```python
from build123d import *

# Parameters (mm, degrees)
BOSS_EXTRUDE1_DEPTH = 31.75
SKETCH5_R           = 6.35
SKETCH5_W           = 31.75
SKETCH5_H           = 19.05
CUT_EXTRUDE1_DEPTH  = 3.302


with BuildPart() as part:
    # Sketch4 → Boss-Extrude1 (new, symmetric)
    with BuildSketch(Plane.XY):
        Polygon((0, 0), (0, 76.2), (3.302, 76.2), (3.302, 3.302), (25.4, 3.302), (25.4, 0), align=None)
    extrude(amount=BOSS_EXTRUDE1_DEPTH, both=True)

    # Sketch5 → Cut-Extrude1 (cut)
    with BuildSketch(Plane(origin=(3.302, 0, 0), x_dir=(0, 0, -1), z_dir=(1, 0, 0))):
        with Locations(Location((0, 57.15, 0), (0, 0, 90))):
            Circle(SKETCH5_R)
        Polygon((-31.75, 63.5), (-31.75, 76.2), (-19.05, 76.2), align=None)
        with Locations((0, 31.75)):
            Rectangle(SKETCH5_W, SKETCH5_H)
        Polygon((19.05, 76.2), (31.75, 63.5), (31.75, 76.2), align=None)
    extrude(amount=-CUT_EXTRUDE1_DEPTH, mode=Mode.SUBTRACT)


solid = part.part
```
The model under review builds one solid part; all positions refer to its coordinate system, in mm. A direction names the side the tool comes from. Coordinates: 2 decimals unless noted, no trailing zeros. Write each loop counter-clockwise with the first axis right and the second up, starting at its lowest first coordinate (ties: lowest second). Pieces come first, ordered by that corner, then holes.
1) We need section D-D on y = 23.5. State the section outline as (x, z) points (3 decimals), then the cut area to 3 significant figures.
2) We need section B-B on z = 0. State the section outline as (x, y) points (3 decimals), then the cut area to 3 significant figures.
3) Machinability: for faces 5 (the face through (2, 41.275, 0)), 6 (the face through (14, 3.302, 0)), 7 (the face through (0, 46, 0)), which of the approach directions +Z, -Z, +X, -X, +Y, -Y give a long, thin tool a straight path to every point of the face, cutting with its end or side? Answer none if there is none.
4) We need section A-A on y = 57.15. State the section outline as (x, z) points.
5) We need section C-C on z = -20.5. State the section outline as (x, y) points, then the cut area to 3 significant figures.
6) Clearance check with a flat-ended pin moving along its axis: pin 1 Ø12 at (y, z) = (33, 18.5) entering from +X. State where the tip first meets the part, or that it passes through.
7) To check wall thickness, follow probe 1 along Z at (x, y) = (1.4, 57.15); probe 2 along X at (y, z) = (49, 5). State the ranges of each line that lie inside material, in increasing order.
8) The part is to be moulded in two halves that separate along Z. For faces 1 (the face through (2, 32, 15.875)), 2 (the face through (1.67, 69.94, -25.31)), 3 (the face through (2, 76.2, 0)), 4 (the face through (2, 32, -15.875)), say which applies: pulls with the +Z half, pulls with the -Z half, needs draft (parallel to the pull), parting line crosses it, or undercut.
Answer list:
1. outline: (0, -31.75) - (3.302, -31.75) - (3.302, -15.875) - (0, -15.875) - close; (0, 15.875) - (3.302, 15.875) - (3.302, 31.75) - (0, 31.75) - close
1. area: 105 mm2
2. outline: (0, 0) - (25.4, 0) - (25.4, 3.302) - (3.302, 3.302) - (3.302, 22.225) - (0, 22.225) - close; (0, 41.275) - (3.302, 41.275) - (3.302, 50.8) - (0, 50.8) - close; (0, 63.5) - (3.302, 63.5) - (3.302, 76.2) - (0, 76.2) - close
2. area: 220 mm2
3. face 5: +X, -X
3. face 6: +Z, -Z, +X, +Y
3. face 7: +Z, -Z, -X, +Y, -Y
4. outline: (0, -31.75) - (3.3, -31.75) - (3.3, -6.35) - (0, -6.35) - close; (0, 6.35) - (3.3, 6.35) - (3.3, 31.75) - (0, 31.75) - close
5. outline: (0, 0) - (25.4, 0) - (25.4, 3.3) - (3.3, 3.3) - (3.3, 74.75) - (0, 74.75) - close
5. area: 320 mm2
6. pin 1: stops at x = 3.3
7. probe 1: z = -31.75 to -6.35, 6.35 to 31.75
7. probe 2: x = 0 to 3.3
8. face 1: undercut
8. face 2: pulls with the -Z half
8. face 3: needs draft
8. face 4: undercut
